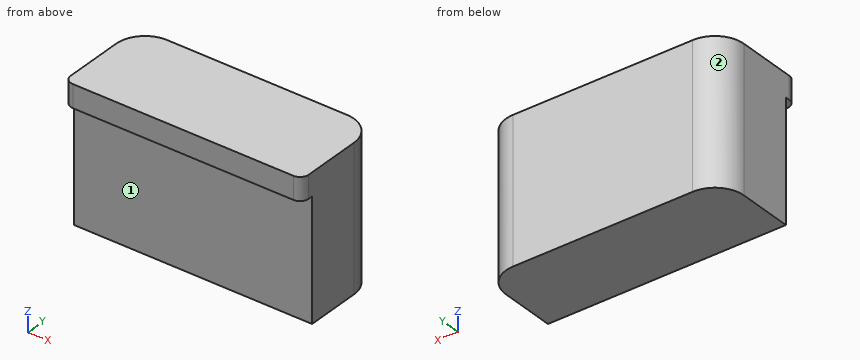
from build123d import *

# Parameters (mm, degrees)
SKETCH1_W           = 8.2
SKETCH1_H           = 3.33
BOSS_EXTRUDE1_DEPTH = 0.785
SKETCH2_W           = 8.2
SKETCH2_H           = 2.88
BOSS_EXTRUDE2_DEPTH = 4.15
FILLET1_R           = 1
FILLET2_R           = 0.3


with BuildPart() as part:
    # Sketch1 → Boss-Extrude1 (new body)
    with BuildSketch(Plane.XY):
        with Locations((0, 1.215)):
            Rectangle(SKETCH1_W, SKETCH1_H)
    extrude(amount=BOSS_EXTRUDE1_DEPTH)

    # Sketch2 → Boss-Extrude2 (add)
    with BuildSketch(Plane(origin=(0, 0, 0), x_dir=(-1, 0, 0), z_dir=(0, 0, -1))):
        with Locations((0, 1.44)):
            Rectangle(SKETCH2_W, SKETCH2_H)
    extrude(amount=BOSS_EXTRUDE2_DEPTH)

    # Fillet1
    fillet1_edges = [part.edges().sort_by_distance(p)[0] for p in [
        (-4.1, 2.88, -1.6825),
        (4.1, 2.88, -1.6825),
    ]]
    fillet(fillet1_edges, radius=FILLET1_R)

    # Fillet2
    fillet2_edges = [part.edges().sort_by_distance(p)[0] for p in [
        (4.1, -0.45, 0.3925),
        (-4.1, -0.45, 0.3925),
    ]]
    fillet(fillet2_edges, radius=FILLET2_R)


solid = part.part
Verification items for the finished model (mm, model axes). Face numbers are marked on the shaded views. A direction names the side the tool comes from. Round coordinates to 2 decimals unless told otherwise and drop trailing zeros. Write each loop counter-clockwise with the first axis right and the second up, starting at its lowest first coordinate (ties: lowest second). Pieces come first, ordered by that corner, then holes.
(1) Section check C-C (y = 2.55). Enter the section's corners in (x, z) (3 decimals), plus the area to 3 significant figures.
Returned:
outline: (-3.842, -4.15) - (3.842, -4.15) - (3.842, 0.785) - (-3.842, 0.785) - close
area: 37.9 mm2
(2) Section check D-D (z = -1.1). Enter the section's corners in (x, y), plus the area to 3 significant figures.
Returned:
outline: (-4.1, 0) - (4.1, 0) - (4.1, 1.88) arc R1 ccw to (3.1, 2.88) - (-3.1, 2.88) arc R1 ccw to (-4.1, 1.88) - close
area: 23.2 mm2
(3) Section check B-B (x = -2.75). Enter the section's corners in (y, z) (3 decimals), plus the area to 3 significant figures.
Returned:
outline: (-0.45, 0) - (0, 0) - (0, -4.15) - (2.88, -4.15) - (2.88, 0.785) - (-0.45, 0.785) - close
area: 14.6 mm2
(4) Material ranges on line 1 (Y direction, x = 1.5, z = -0.15); line 2 (Z direction, x = 1, y = -0.15) (3 decimals); line 3 (Y direction, x = 3.5, z = -1.55), recorded low to high.
Returned:
line 1: y = 0 to 2.88
line 2: z = 0 to 0.785
line 3: y = 0 to 2.8
(5) Section check A-A (z = 0.4). Enter the section's corners in (x, y).
Returned:
outline: (-4.1, -0.15) arc R0.3 ccw to (-3.8, -0.45) - (3.8, -0.45) arc R0.3 ccw to (4.1, -0.15) - (4.1, 1.88) arc R1 ccw to (3.1, 2.88) - (-3.1, 2.88) arc R1 ccw to (-4.1, 1.88) - close
(6) Access from +Z, -Z, +X, -X, +Y, -Y to the whole of each face (thin tool, end or side, straight path). Record for the marked faces 1 and 2.
Returned:
face 1: -Z, +X, -X, -Y
face 2: +Z, -Z, -X, +Y
